The listing builds one solid part. Answer for the finished solid, in the listing's coordinates (mm). A direction names the side the tool comes from. Give positions to 0.01 mm unless a question says otherwise; leave off trailing zeros. Write each loop counter-clockwise with the first axis right and the second up, starting at its lowest first coordinate (ties: lowest second). Pieces come first, ordered by that corner, then holes. Notation, with made-up numbers: (21.5, 79.25) -> (41.5, 79.25) arc R20 cw to (41.5, 93.25) -> close; hole circle Ø5 at (45.5, -31.5). An arc over 180 degrees is marked (long way). Put each result on its own line as item: value. Start each with the question number.
1) Flat-ended cylindrical pins translate along their axes: pin 1 Ø18 at (x, y) = (55, 55) entering from +Z; pin 2 Ø4 at (x, z) = (72.5, 39.5) entering from +Y; pin 3 Ø5 at (x, y) = (89, 21) entering from +Z; pin 4 Ø12 at (y, z) = (12, 30.5) entering from +X. Find the tip coordinate at first contact, or state that the pin passes through.
2) For faces 4 (the flat face through (70, 18, 13)), 5 (the flat face through (54.23, 4.93, 2.535)), determine the directions among +Z, -Z, +X, -X, +Y, -Y from which every point of the face is accessible in a straight line to the end or side of a thin tool.
3) Find the intervals of material crossed by line 1 along X through (y, z) = (36, 15.5); line 2 along Y through (x, z) = (55, 8.25); line 3 along Y through (x, z) = (63, 38), in increasing order. Write a range as from..to.
4) A cutting plane is placed at D-D (x = 92). Write down the section's boundary in (y, z), then the cut area to 3 significant figures.
5) A cutting plane is placed at B-B (y = 55). Write down the section's boundary in (x, z), then the cut area to 3 significant figures.
6) For a pull along X with two mould halves and no side action, classify faces 1 (the flat face through (32.25, 55, 30)), 2 (the flat face through (54, 110, 12)), 3 (the flat face through (18, 40, 13)) as released by +X, released by -X, zero draft, split by the parting line, or undercut.
7) A cutting plane is placed at A-A (z = 24). Write down the section's boundary in (x, y), then the cut area to 3 significant figures.
from build123d import *

# Parameters (mm, degrees)
F0_W      = 110
F0_H      = 110
F1_DEPTH  = 20
F2_W      = 30
F2_H      = 18.75
F2_W_2    = 18.75
F2_H_2    = 30
F3_DEPTH  = 5
F2_W_3    = 45.5
F2_H_3    = 45.5
F4_DEPTH  = 30
F2_R      = 4.5
F5_DEPTH  = 20.001
F2_R_2    = 10
F6_DEPTH  = 10
F7_SIZE2  = 5
F7_SIZE   = 10
F8_SIZE   = 1
F9_DEPTH  = 10
F10_DEPTH = 15


with BuildPart() as f1:
    # F0 (on Top) → F1 (new body)
    with BuildSketch(Plane.XY):
        with Locations((55, 55)):
            Rectangle(F0_W, F0_H)
    extrude(amount=F1_DEPTH)

    # F2 (on face) → F3 (cut)
    with BuildSketch(Plane.XY.offset(20)):
        Polygon((27.25, 70), (27.25, 82.75), (40, 82.75), (40, 101.5), (8.5, 101.5), (8.5, 70), align=None)
        with Locations((55, 92.125)):
            Rectangle(F2_W, F2_H)
        Polygon((70, 101.5), (70, 82.75), (82.75, 82.75), (82.75, 70), (101.5, 70), (101.5, 101.5), align=None)
        with Locations((92.125, 55)):
            Rectangle(F2_W_2, F2_H_2)
        with Locations((55, 17.875)):
            Rectangle(F2_W, F2_H)
        with Locations((17.875, 55)):
            Rectangle(F2_W_2, F2_H_2)
    extrude(amount=-F3_DEPTH, mode=Mode.SUBTRACT)

    # F2 (on face) → F4 (join)
    with BuildSketch(Plane.XY.offset(20)):
        Polygon((40, 82.75), (27.25, 82.75), (27.25, 70), (27.25, 40), (27.25, 27.25), (40, 27.25), (70, 27.25), (82.75, 27.25), (82.75, 40), (82.75, 70), (82.75, 82.75), (70, 82.75), align=None)
        with Locations((55, 55)):
            Rectangle(F2_W_3, F2_H_3, mode=Mode.SUBTRACT)
    extrude(amount=F4_DEPTH)

    # F2 (on face) → F5 (cut, through all)
    with BuildSketch(Plane.XY.offset(20)):
        with Locations((55, 55)):
            Circle(F2_R)
    extrude(amount=-F5_DEPTH, mode=Mode.SUBTRACT)

    # F2 (on face) → F6 (cut)
    with BuildSketch(Plane.XY.offset(20)):
        with Locations((55, 55)):
            Rectangle(F2_W_3, F2_H_3)
        with Locations((55, 55)):
            Circle(F2_R_2, mode=Mode.SUBTRACT)
    extrude(amount=-F6_DEPTH, mode=Mode.SUBTRACT)

    # F7
    f7_edges = [f1.edges().sort_by_distance(p)[0] for p in [
        (55, 110, 0),
        (0, 55, 0),
        (55, 0, 0),
        (110, 55, 0),
    ]]
    f7_side = f1.faces().sort_by_distance((1.555635, 55, 0))[0]
    chamfer(f7_edges, length=F7_SIZE, length2=F7_SIZE2, reference=f7_side)

    # F8
    f8_edges = [f1.edges().sort_by_distance(p)[0] for p in [
        (55, 27.25, 50),
        (27.25, 55, 50),
        (82.75, 55, 50),
        (55, 82.75, 50),
    ]]
    chamfer(f8_edges, length=F8_SIZE)

    # F2 (on face) → F9 (cut)
    with BuildSketch(Plane.XY.offset(20)):
        Polygon((27.25, 70), (27.25, 82.75), (40, 82.75), (40, 101.5), (8.5, 101.5), (8.5, 70), align=None)
        Polygon((27.25, 27.25), (27.25, 40), (8.5, 40), (8.5, 8.5), (40, 8.5), (40, 27.25), align=None)
        Polygon((101.5, 40), (82.75, 40), (82.75, 27.25), (70, 27.25), (70, 8.5), (101.5, 8.5), align=None)
        Polygon((70, 101.5), (70, 82.75), (82.75, 82.75), (82.75, 70), (101.5, 70), (101.5, 101.5), align=None)
    extrude(amount=-F9_DEPTH, mode=Mode.SUBTRACT)

    # F2 (on face) → F10 (cut)
    with BuildSketch(Plane.XY.offset(20)):
        with Locations((55, 55)):
            Circle(F2_R_2)
        with Locations((55, 55)):
            Circle(F2_R, mode=Mode.SUBTRACT)
    extrude(amount=-F10_DEPTH, mode=Mode.SUBTRACT)


solid = f1.part
Reply:
1. pin 1: stops at z = 5
1. pin 2: stops at y = 82.75
1. pin 3: stops at z = 10
1. pin 4: passes through
2. face 4: +Z
2. face 5: -Z, +X, -X, -Y
3. line 1: x = 0..8.5, 27.25..32.25, 77.75..82.75, 101.5..110
3. line 2: y = 0..45, 65..110
3. line 3: y = 27.25..32.25, 77.75..82.75
4. outline: (0, 5) -> (10, 0) -> (100, 0) -> (110, 5) -> (110, 20) -> (101.5, 20) -> (101.5, 10) -> (70, 10) -> (70, 15) -> (40, 15) -> (40, 10) -> (8.5, 10) -> (8.5, 20) -> (0, 20) -> close
4. area: 1,370 mm2
5. outline: (0, 5) -> (10, 0) -> (50.5, 0) -> (50.5, 5) -> (45, 5) -> (45, 10) -> (32.25, 10) -> (32.25, 50) -> (28.25, 50) -> (27.25, 49) -> (27.25, 15) -> (8.5, 15) -> (8.5, 20) -> (0, 20) -> close; (59.5, 0) -> (100, 0) -> (110, 5) -> (110, 20) -> (101.5, 20) -> (101.5, 15) -> (82.75, 15) -> (82.75, 49) -> (81.75, 50) -> (77.75, 50) -> (77.75, 10) -> (65, 10) -> (65, 5) -> (59.5, 5) -> close
5. area: 1,660 mm2
6. face 1: undercut
6. face 2: zero draft
6. face 3: undercut
7. outline: (27.25, 27.25) -> (82.75, 27.25) -> (82.75, 82.75) -> (27.25, 82.75) -> close; hole (32.25, 32.25) -> (77.75, 32.25) -> (77.75, 77.75) -> (32.25, 77.75) -> close
7. area: 1,010 mm2
